from build123d import *

# Parameters (mm, degrees)
EXTRUDE_1_DEPTH = 3


with BuildPart() as part:
    # Sketch 273 → Бобышка-Вытянуть1 (new body)
    with BuildSketch(Plane.XY):
        Polygon((148.354716995, -23.671565122), (40.597138959, -57.662313559), (-40.597138959, -57.662313559), (-148.354716995, -23.671565122), (-162, -18.92), (-152.5, 58), (-58.64, 58), (0, 38.59), (58.64, 58), (152.5, 58), (162, -18.92), align=None)
        with BuildLine():
            Line((-10.908195141, 11.626317085), (-21.848195141, 15.513282482))
            Line((-21.848195141, 15.513282482), (-18.617591482, 3.873282482))
            ThreePointArc((-18.617591482, 3.873282482), (0, -28.455), (18.617591482, 3.873282482))
            Line((18.617591482, 3.873282482), (21.848195141, 15.513282482))
            Line((21.848195141, 15.513282482), (10.908195141, 11.626317085))
            ThreePointArc((10.908195141, 11.626317085), (0, 14.595), (-10.908195141, 11.626317085))
        make_face(mode=Mode.SUBTRACT)
    extrude(amount=EXTRUDE_1_DEPTH)


solid = part.part
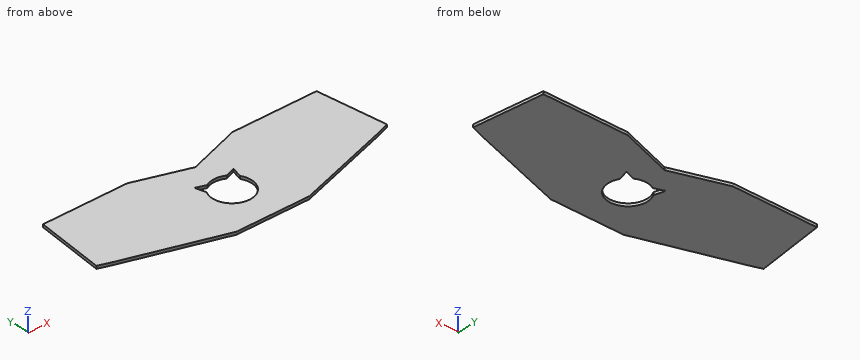
Could you check a few things on this model? Use its own coordinates, in mm. Round coordinates to 2 decimals unless told otherwise and drop trailing zeros. Order: outer loops, then holes, each group sorted by start corner. A loop starts at its lowest first (then second) coordinate and runs counter-clockwise, first axis right, second up.
(1) Imagine slicing it at B-B (z = 1.85). Write out the boundary of the cut face in (x, y) (3 decimals).
Response values:
outline: (-162, -18.92) - (-148.355, -23.672) - (-40.597, -57.662) - (40.597, -57.662) - (148.355, -23.672) - (162, -18.92) - (152.5, 58) - (58.64, 58) - (0, 38.59) - (-58.64, 58) - (-152.5, 58) - close; hole (-21.848, 15.513) - (-18.618, 3.873) arc R21.525 ccw (long way) to (18.618, 3.873) - (21.848, 15.513) - (10.908, 11.626) arc R21.525 ccw to (-10.908, 11.626) - close
(2) Imagine slicing it at A-A (y = -6.93). Write out the boundary of the cut face in (x, z) (3 decimals).
Response values:
outline: (-160.519, 0) - (-21.525, 0) - (-21.525, 3) - (-160.519, 3) - close; (21.525, 0) - (160.519, 0) - (160.519, 3) - (21.525, 3) - close
(3) Imagine slicing it at C-C (x = 8). Write out the boundary of the cut face in (y, z), plus the area to 3 significant figures.
Response values:
outline: (-57.66, 0) - (-26.91, 0) - (-26.91, 3) - (-57.66, 3) - close; (13.05, 0) - (41.24, 0) - (41.24, 3) - (13.05, 3) - close
area: 177 mm2
(4) Please list where these lines run through material, in increasing order: line 1 along X through (y, z) = (-6.93, 1.9) (3 decimals); line 2 along Y through (x, z) = (-72, 2.75); line 3 along Y through (x, z) = (-57, 2.2).
Response values:
line 1: x = -160.519 to -21.525, 21.525 to 160.519
line 2: y = -47.76 to 58
line 3: y = -52.49 to 57.46
(5) I'm going to push a flat-ended pin straight in: pin 1 (1 mm diameter, centred on x = 87.5, z = 1.5, fed in from -Y). Where does the tip first touch, or does it pass through?
Response values:
pin 1: stops at y = -43.03
(6) Imagine slicing it at D-D (y = 29.5). Write out the boundary of the cut face in (x, z), plus the area to 3 significant figures.
Response values:
outline: (-156.02, 0) - (156.02, 0) - (156.02, 3) - (-156.02, 3) - close
area: 936 mm2
